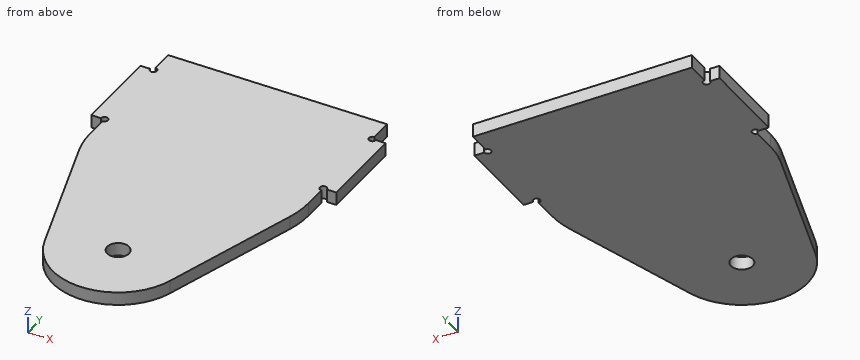
```python
from build123d import *

# Parameters (mm, degrees)
SKETCH1_W           = 50
SKETCH1_H           = 35
SKETCH1_R           = 2.5
BOSS_EXTRUDE1_DEPTH = 3
FILLET1_R           = 20
SKETCH2_W           = 6
SKETCH2_H           = 20
BOSS_EXTRUDE2_DEPTH = 3
SKETCH3_R           = 0.8
CUT_EXTRUDE1_DEPTH  = 69.551075849


with BuildPart() as part:
    # Sketch1 → Boss-Extrude1 (new body)
    # profile 1 of 2: a face of its own
    with BuildSketch(Plane.XY):
        Rectangle(SKETCH1_W, SKETCH1_H)
    # profile 2 of 2: a face of its own
    with BuildSketch(Plane.XY):
        with BuildLine():
            Line((-25, -17.5), (-14.327856223, -51.939880186))
            ThreePointArc((-14.327856223, -51.939880186), (0, -62.5), (14.327856223, -51.939880186))
            Line((14.327856223, -51.939880186), (25, -17.5))
            Line((25, -17.5), (-25, -17.5))
        make_face()
        with Locations((0, -47.5)):
            Circle(SKETCH1_R, mode=Mode.SUBTRACT)
    extrude(amount=BOSS_EXTRUDE1_DEPTH)

    # Fillet1
    fillet1_edges = [part.edges().sort_by_distance(p)[0] for p in [
        (25, -17.5, 1.5),
        (-25, -17.5, 1.5),
    ]]
    fillet(fillet1_edges, radius=FILLET1_R)

    # Sketch2 → Boss-Extrude2 (add)
    with BuildSketch(Plane.XY.offset(3)):
        with Locations((-25, 1.513878189)):
            Rectangle(SKETCH2_W, SKETCH2_H)
        with Locations((25, 1.513878189)):
            Rectangle(SKETCH2_W, SKETCH2_H)
    extrude(amount=-BOSS_EXTRUDE2_DEPTH)

    # Sketch3 → Cut-Extrude1 (cut, through all)
    with BuildSketch(Plane.XY.offset(3)):
        with Locations((-25, 11.513878189)):
            Circle(SKETCH3_R)
        with Locations((-25, -8.486121811)):
            Circle(SKETCH3_R)
        with Locations((25, 11.513878189)):
            Circle(SKETCH3_R)
        with Locations((25, -8.486121811)):
            Circle(SKETCH3_R)
    extrude(amount=-CUT_EXTRUDE1_DEPTH, mode=Mode.SUBTRACT)


solid = part.part
```
For this review, take the finished solid that the model builds, in its own axes (mm). Give positions to 0.01 mm unless a question says otherwise; leave off trailing zeros. Loops run counter-clockwise (first coordinate to the right, second up) from the corner with the lowest first, then second, coordinate; pieces in that order, holes last. Notation, with made-up numbers: M 86,41 L 133,41 A29 ccw 133,72 Z; hole C -38.75,73 d4. An arc over 180 degrees is marked long. One line per item, written item: value. Start each with the question number.
Q1. Add section B-B (x = 0). Give the boundary of the cut face in (y, z).
Q2. Add section C-C (y = -47.5). Give the boundary of the cut face in (x, z), and give its area (3 significant figures).
Q3. Add section D-D (y = -11). Give the boundary of the cut face in (x, z), and give its area (3 significant figures).
Q4. For L1, parallel to Y at x = 0, z = 2.3; L2, parallel to X at y = -15, z = 2.85; L3, parallel to X at y = -48, z = 1.3, list the stretches that pass through material, from the lowest coordinate up.
Q5. Clearance check with flat-ended pins moving along their axes: pin 1 Ø1.5 at (y, z) = (-24.5, 1) entering from -X; pin 2 Ø1.5 at (y, z) = (-13, 2) entering from -X; pin 3 Ø1.1 at (x, z) = (-27.5, 1.5) entering from -Y. State where each tip first meets the part, or that it passes through.
Q6. Add section A-A (z = 1.45). Give the boundary of the cut face in (x, y).
Reply:
1. outline: M -62.5,0 L -50,0 L -50,3 L -62.5,3 Z; M -45,0 L 17.5,0 L 17.5,3 L -45,3 Z
2. outline: M -15.7,0 L -2.5,0 L -2.5,3 L -15.7,3 Z; M 2.5,0 L 15.7,0 L 15.7,3 L 2.5,3 Z
2. area: 79.2 mm²
3. outline: M -25,0 L 25,0 L 25,3 L -25,3 Z
3. area: 150 mm²
4. L1: -62.5 to -50, -45 to 17.5
4. L2: -24.99 to 24.99
4. L3: -15.55 to -2.45, 2.45 to 15.55
5. pin 1: x = -23.06
5. pin 2: x = -25
5. pin 3: y = -8.49
6. outline: M -28,-8.49 L -25.8,-8.49 A0.8 cw long -25,-9.29 L -25,-14.47 A20 ccw -24.1,-20.39 L -14.33,-51.94 A15 ccw 14.33,-51.94 L 24.1,-20.39 A20 ccw 25,-14.47 L 25,-9.29 A0.8 cw long 25.8,-8.49 L 28,-8.49 L 28,11.51 L 25.8,11.51 A0.8 cw long 25,12.31 L 25,17.5 L -25,17.5 L -25,12.31 A0.8 cw long -25.8,11.51 L -28,11.51 Z; hole C 0,-47.5 d5
